```python
from build123d import *

# Parameters (mm, degrees)
F0_W     = 101.6
F0_H     = 63.5
F1_DEPTH = 76.2
F3_DEPTH = 63.5
F5_DEPTH = 50.8


with BuildPart() as f1:
    # F0 (on Front) → F1 (new body)
    with BuildSketch(Plane.XZ):
        with Locations((-1.3990358829, -7.4705901444)):
            Rectangle(F0_W, F0_H)
    extrude(amount=F1_DEPTH)

    # F2 (on face) → F3 (cut)
    with BuildSketch(Plane.XY.offset(24.2794098556)):
        with BuildLine():
            Line((49.4009641171, -63.5), (49.4009641171, -12.7))
            ThreePointArc((49.4009641171, -12.7), (24.0009641171, -38.1), (49.4009641171, -63.5))
        make_face()
    extrude(amount=-F3_DEPTH, mode=Mode.SUBTRACT)

    # F4 (on face) → F5 (cut)
    with BuildSketch(Plane(origin=(-52.1990358829, 0, 0), x_dir=(0, -1, 0), z_dir=(-1, 0, 0))):
        with BuildLine():
            Line((76.2, 24.2794098556), (25.4, 24.2794098556))
            ThreePointArc((25.4, 24.2794098556), (40.8007490362, -11.1198411082), (76.2, -26.5205901444))
            Line((76.2, -26.5205901444), (76.2, 24.2794098556))
        make_face()
    extrude(amount=-F5_DEPTH, mode=Mode.SUBTRACT)


solid = f1.part
```
CAD build for the part. Positions are in the model's coordinates, mm. A direction names the side the tool comes from. Coordinates: 2 decimals unless noted, no trailing zeros. Order: outer loops, then holes, each group sorted by start corner. A loop starts at its lowest first (then second) coordinate and runs counter-clockwise, first axis right, second up.
(1) Saw through at D-D, the plane y = -37. Write the cut outline in (x, z), and give its area (3 significant figures).
Solution:
outline: (-52.2, -39.22) - (24.02, -39.22) - (24.02, 24.28) - (-1.4, 24.28) - (-1.4, -6.88) - (-52.2, -6.88) - close
area: 3,260 mm2
(2) Which spindle directions (+Z, -Z, +X, -X, +Y, -Y) get a long thin tool onto all of the face, cutting with end or side? Do faces 4 (the face through (-1.399, -56, 5)), 5 (the face through (-52.199, -29, -15)). Say none if no direction does.
Solution:
face 4: +Z, -X, -Y
face 5: +Z, -Z, -X, +Y, -Y
(3) Saw through at A-A, the plane x = 35. Write the cut outline in (y, z).
Solution:
outline: (-76.2, -39.22) - (-59.02, -39.22) - (-59.02, 24.28) - (-76.2, 24.28) - close; (-17.18, -39.22) - (0, -39.22) - (0, 24.28) - (-17.18, 24.28) - close
(4) Saw through at C-C, the plane x = -19.5. Write the cut outline in (y, z), and give its area (3 significant figures).
Solution:
outline: (-76.2, -39.22) - (0, -39.22) - (0, 24.28) - (-25.4, 24.28) arc R52.69 cw to (-76.2, -26.52) - close
area: 2,850 mm2
(5) Saw through at B-B, the plane z = -13.5. Write the cut outline in (x, y), and give its area (3 significant figures).
Solution:
outline: (-52.2, -43.34) - (-1.4, -43.34) - (-1.4, -76.2) - (49.4, -76.2) - (49.4, -63.5) arc R25.4 cw to (49.4, -12.7) - (49.4, 0) - (-52.2, 0) - close
area: 5,060 mm2
(6) Mould opens along Y. For faces 1 (the face through (24, -38, -7)), 2 (the face through (49.401, -6, -8)), 3 (the face through (-27.155, -40.412, -10.727)) say: released by +Y, released by -Y, zero draft, split by the parting line, or undercut.
Solution:
face 1: undercut
face 2: zero draft
face 3: released by -Y
(7) Pin check, flat tips, straight feed: pin 1 Ø3 at (y, z) = (-49.5, 17) entering from -X; pin 2 Ø1 at (y, z) = (-24.5, 11) entering from +X; pin 3 Ø12 at (y, z) = (-39.5, -3) entering from +X. Stop position of each tip, or through.
Solution:
pin 1: stops at x = -1.4
pin 2: stops at x = 28.27
pin 3: stops at x = 25.1
(8) Drill centre lines: L1, parallel to Y at x = 30, z = -20; L2, parallel to Y at x = 28.5, z = 0.5; L3, parallel to Y at x = -5, z = -5.5. Where is each one in solid material? Low to high.
Solution:
L1: y = -76.2 to -54.49, -21.71 to 0
L2: y = -76.2 to -52.53, -23.67 to 0
L3: y = -35.92 to 0
